The drawing under review shows one solid part. Ordinate dimensions are in mm from its lowest x, y, z. A direction names the side the tool comes from. Coordinates: 2 decimals unless noted, no trailing zeros. Loops run counter-clockwise (first coordinate to the right, second up) from the corner with the lowest first, then second, coordinate; pieces in that order, holes last. Notation, with made-up numbers: M 73.5,-37 L 95.5,-37 A19 cw 95.5,-26 Z; hole C -8.75,-13.5 d10. An arc over 180 degrees is marked long. Return JSON: item names as keys, results as strings.
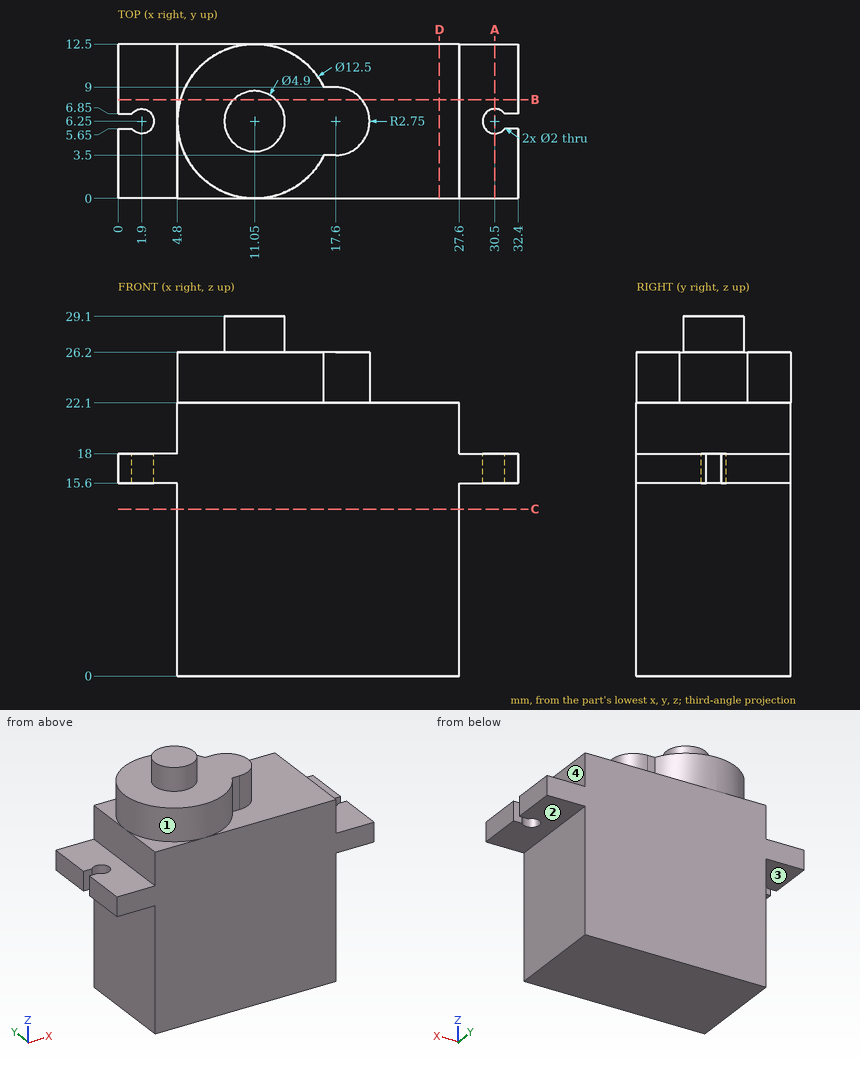
1. Insertion check: pin 1 Ø2.5 at (x, y) = (30.5, 4.5) entering from -Z; pin 2 Ø1.2 at (x, y) = (1.9, 6.25) entering from +Z; pin 3 Ø3 at (y, z) = (9, 14) entering from -X; pin 4 Ø1 at (x, y) = (23, 2) entering from +Z. Each pin has a flat end and moves straight along its axis. Give the tip position at first contact, or say it passes through.
Check values:
{"pin 1": "z = 15.6", "pin 2": "through", "pin 3": "x = 4.8", "pin 4": "z = 22.1"}
2. Machinability: for the marked faces 1, 2, 3 and 4, which of the approach directions +Z, -Z, +X, -X, +Y, -Y give a long, thin tool a straight path to every point of the face, cutting with its end or side? Answer none if there is none.
Check values:
{"face 1": "+Z", "face 2": "-Z, +X, +Y, -Y", "face 3": "-Z, -X, +Y, -Y", "face 4": "+Z, +X, +Y, -Y"}
3. Add section D-D on x = 26. Give the boundary of the cut face in (y, z).
Check values:
{"outline": "M 0,0 L 12.5,0 L 12.5,22.1 L 0,22.1 Z"}
4. Add section C-C on z = 13.5. Give the boundary of the cut face in (x, y).
Check values:
{"outline": "M 4.8,0 L 27.6,0 L 27.6,12.5 L 4.8,12.5 Z"}
5. Add section B-B on y = 8. Give the boundary of the cut face in (x, z), plus the area to 3 significant figures.
Check values:
{"outline": "M 0,15.6 L 4.8,15.6 L 4.8,0 L 27.6,0 L 27.6,15.6 L 32.4,15.6 L 32.4,18 L 27.6,18 L 27.6,22.1 L 19.72,22.1 L 19.72,26.2 L 12.76,26.2 L 12.76,29.1 L 9.34,29.1 L 9.34,26.2 L 5.05,26.2 L 5.05,22.1 L 4.8,22.1 L 4.8,18 L 0,18 Z", "area": "597 mm²"}
6. Add section A-A on x = 30.5. Give the boundary of the cut face in (y, z).
Check values:
{"outline": "M 0,15.6 L 5.25,15.6 L 5.25,18 L 0,18 Z; M 7.25,15.6 L 12.5,15.6 L 12.5,18 L 7.25,18 Z"}
7. To check wall thickness, follow line 1 (Y direction, x = 1.9, z = 16.2); line 2 (X direction, y = 5, z = 14.75); line 3 (Z direction, x = 12, y = 3.5). State the ranges of each line that lie inside material, in increasing order.
Check values:
{"line 1": "0 to 5.25, 7.25 to 12.5", "line 2": "4.8 to 27.6", "line 3": "0 to 26.2"}
